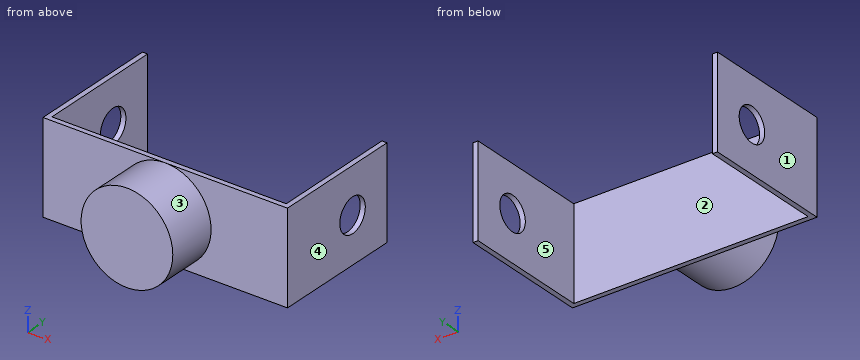
Autodesk Inventor part; units mm, degrees
ref_plane "YZ Plane" through (0, 0, 0) normal (1, 0, 0) x (0, 1, 0)
ref_plane "XZ Plane" through (0, 0, 0) normal (0, 1, 0) x (-1, 0, 0)
ref_plane "XY Plane" through (0, 0, 0) normal (0, 0, 1) x (1, 0, 0)
sketch "Sketch1" plane through (0, 0, 0) normal (0, 0, 1) x (1, 0, 0)
  line L0 (0, 0) -> (27, 0) construction
  line L1 (27, 0) -> (27, 27)
  line L2 (27, 27) -> (0, 27)
  line L3 (0, 27) -> (0, 0) construction
  line L4 (-27, 0) -> (-27, 27)
  line L5 (-27, 27) -> (0, 27)
  line L6 (27, 0) -> (27, -27)
  line L7 (27, -27) -> (0, -27)
  line L8 (-27, -27) -> (0, -27)
  line L9 (-27, 0) -> (-27, -27)
  dimension "d0" = 27
extrude "Extrusion1" add sketch "Sketch1" along normal mid plane 138
sketch "Sketch2" plane through (0, 0, 69) normal (0, 0, 1) x (1, 0, 0)
  line L0 (27, -27) -> (27, 27)
  line L1 (27, 27) -> (-27, 27)
  line L2 (-27, 27) -> (-27, -27)
  line L3 (-27, -27) -> (27, -27)
  circle A0 centre (0, 0) radius 27
extrude "Extrusion2" cut sketch "Sketch2" against normal blind 30 contours L3 A0 L0 | A0 L1 L0 | L3 L2 A0 | A0 L2 L1
sketch "Sketch3" plane through (0, 0, 69) normal (0, 0, 1) x (1, 0, 0)
  circle A0 centre (0, 0) radius 27
  line L0 (-51, 27) -> (27, 27)
  line L1 (27, 27) -> (27, -27)
  line L2 (27, -27) -> (-51, -27)
  line L3 (-51, -27) -> (-51, 27)
  line L4 (27, 27) -> (27, 0)
  line L5 (27, 27) -> (27, -27)
  line L6 (0, 27) -> (27, 27)
  line L7 (27, -27) -> (0, -27)
  dimension "d6" = 51
extrude "Extrusion3" add sketch "Sketch3" along normal blind 3
sketch "Sketch4" plane through (0, 0, 72) normal (0, 0, 1) x (1, 0, 0)
  circle A0 centre (0, 0) radius 10
  dimension "d9" = 20
extrude "Extrusion4" cut sketch "Sketch4" against normal blind 3
mirror "Mirror1" about plane through (0, 0, 0) normal (0, 0, 1) of "Extrusion3", "Extrusion4"
sketch "Sketch5" plane through (-51, 27, -69) normal (0, 0, 1) x (1, 0, 0)
  line L0 (24, -54) -> (0, -54)
  line L1 (0, 0) -> (3, 0)
  line L2 (3, 0) -> (3, -54)
  line L3 (3, -54) -> (0, -54)
  line L4 (0, -54) -> (0, 0)
  point P0 (51, -27)
  dimension "d13" = 3
extrude "Extrusion5" add sketch "Sketch5" along normal up to next
sketch "Sketch6" plane through (-51, -27, 72) normal (-1, 0, 0) x (0, 0, 1)
  line L0 (0, 0) -> (-144, 0)
  circle A0 centre (-72, 27) radius 27
extrude "Extrusion6" add sketch "Sketch6" along normal blind 30
sketch "Sketch7" plane through (-27, 27, 39) normal (0, 1, 0) x (1, 0, 0)
  line L0 (0, 108) -> (54, 108)
  line L1 (54, 108) -> (54, -30)
  line L2 (54, -30) -> (0, -30)
  line L3 (0, -30) -> (0, 108)
  point P0 (27, 39)
extrude "Extrusion7" cut sketch "Sketch7" against normal through all
move or copy body "Move Body1" bodies to move or copy 1 copy no rotation origin (0, 0, 0) rotation axis (1, 0, 0) rotation angle 90
move or copy body "Move Body2" bodies to move or copy 1 copy no rotation origin (0, 0, 0) rotation axis (0, 0, 1) rotation angle 90
properties part number "Sholder_Pitch"
Can you work these out from the model? Positions are in its coordinate system, mm. Face numbers are marked on the shaded views. A direction names the side the tool comes from. Give positions to 0.01 mm unless a question says otherwise; leave off trailing zeros. Loops run counter-clockwise (first coordinate to the right, second up) from the corner with the lowest first, then second, coordinate; pieces in that order, holes last. Notation, with made-up numbers: (14, 78.25) -> (52, 78.25) arc R10 ccw to (52, 97.25) -> close; hole circle Ø5 at (20, 0.25). An arc over 180 degrees is marked (long way). Write item = value, one per line.
1) Suppose I cut it at D-D on z = 16. Write out the boundary of the cut face in (x, y), then the cut area to 3 significant figures.
Check result:
outline = (-72, -51) -> (-21.75, -51) -> (-21.75, -81) -> (21.75, -81) -> (21.75, -51) -> (72, -51) -> (72, 27) -> (69, 27) -> (69, -48) -> (-69, -48) -> (-69, 27) -> (-72, 27) -> close
area = 2,190 mm2
2) Thinking about a two-plate mould opening in X: for the marked faces 3, 4 and 5, which applies, released by +X, released by -X, zero draft, split by the parting line, or undercut?
Check result:
face_3 = split by the parting line
face_4 = released by +X
face_5 = undercut
3) Suppose I cut it at B-B on y = 19. Write out the boundary of the cut face in (x, z).
Check result:
outline = (-72, -27) -> (-69, -27) -> (-69, 27) -> (-72, 27) -> close; (69, -27) -> (72, -27) -> (72, 27) -> (69, 27) -> close
4) Suppose I cut it at C-C on y = 0. Write out the boundary of the cut face in (x, z).
Check result:
outline = (-72, -27) -> (-69, -27) -> (-69, -10) -> (-72, -10) -> close; (-72, 10) -> (-69, 10) -> (-69, 27) -> (-72, 27) -> close; (69, -27) -> (72, -27) -> (72, -10) -> (69, -10) -> close; (69, 10) -> (72, 10) -> (72, 27) -> (69, 27) -> close
5) Will these pins go through, and if not, where does the flat tip stop? pin 1 (12 mm diameter, centred on y = 0, z = 0, fed in from +X); pin 2 (10 mm diameter, centred on x = 55.5, z = 19, fed in from +Y); pin 3 (1 mm diameter, centred on y = -65, z = 11, fed in from -X); pin 4 (2 mm diameter, centred on x = -37, z = -12, fed in from -Y).
Check result:
pin_1 = through
pin_2 = -48
pin_3 = -24.87
pin_4 = -51
6) I need wall thicknesses on L1, parallel to Z at x = -69.8, y = 0; L2, parallel to X at y = 6, z = -18; L3, parallel to Y at x = -63.5, z = 21.5. Which ranges of each line are inside material? Lowest first, please. Write a range as from..to.
Check result:
L1 = -27..-10, 10..27
L2 = -72..-69, 69..72
L3 = -51..-48
7) Suppose I cut it at A-A on z = 0. Write out the boundary of the cut face in (x, y), then the cut area to 3 significant figures.
Check result:
outline = (-72, -51) -> (-27, -51) -> (-27, -81) -> (27, -81) -> (27, -51) -> (72, -51) -> (72, -10) -> (69, -10) -> (69, -48) -> (-69, -48) -> (-69, -10) -> (-72, -10) -> close; (-72, 10) -> (-69, 10) -> (-69, 27) -> (-72, 27) -> close; (69, 10) -> (72, 10) -> (72, 27) -> (69, 27) -> close
area = 2,380 mm2
8) For the marked faces 1 and 2, which set-ups out of +Z, -Z, +X, -X, +Y, -Y let a thin tool reach every point of the face, with its end or its side?
Check result:
face_1 = +Z, -Z, -X, +Y, -Y
face_2 = +Z, -Z, +Y
